from build123d import *

# Parameters (mm, degrees)
F0_W     = 20.5
F0_H     = 4.5
F1_DEPTH = 5
F2_DEPTH = 5
F3_R     = 3
F4_R     = 0.5
F5_DEPTH = 3


with BuildPart() as f1:
    # F0 (on Top) → F1 (new body)
    with BuildSketch(Plane.XY):
        with BuildLine():
            ThreePointArc((4.5, 2.1794494718), (0, -5), (-4.5, 2.1794494718))
            Line((-4.5, 2.1794494718), (-10.5, 2.1794494718))
            Line((-10.5, 2.1794494718), (-11.5394689808, -2.1748499468))
            Line((-11.5394689808, -2.1748499468), (-2, -10))
            Line((-2, -10), (-13.4075078933, -10))
            Line((-13.4075078933, -10), (-16.3915383908, -22.5))
            Line((-16.3915383908, -22.5), (16.3915383908, -22.5))
            Line((16.3915383908, -22.5), (13.4075078933, -10))
            Line((13.4075078933, -10), (2, -10))
            Line((2, -10), (11.5394689808, -2.1748499468))
            Line((11.5394689808, -2.1748499468), (10.5, 2.1794494718))
            Line((10.5, 2.1794494718), (4.5, 2.1794494718))
        make_face()
        with Locations((0, -16.25)):
            Rectangle(F0_W, F0_H, mode=Mode.SUBTRACT)
        with BuildLine():
            Line((4.5, 2.1794494718), (-4.5, 2.1794494718))
            ThreePointArc((-4.5, 2.1794494718), (0, -5), (4.5, 2.1794494718))
        make_face()
    extrude(amount=-F1_DEPTH)

    # F0 (on Top) → F2 (join)
    with BuildSketch(Plane.XY):
        with BuildLine():
            ThreePointArc((4.5, 2.1794494718), (0, -5), (-4.5, 2.1794494718))
            Line((-4.5, 2.1794494718), (-10.5, 2.1794494718))
            Line((-10.5, 2.1794494718), (-11.5394689808, -2.1748499468))
            Line((-11.5394689808, -2.1748499468), (-2, -10))
            Line((-2, -10), (-13.4075078933, -10))
            Line((-13.4075078933, -10), (-16.3915383908, -22.5))
            Line((-16.3915383908, -22.5), (16.3915383908, -22.5))
            Line((16.3915383908, -22.5), (13.4075078933, -10))
            Line((13.4075078933, -10), (2, -10))
            Line((2, -10), (11.5394689808, -2.1748499468))
            Line((11.5394689808, -2.1748499468), (10.5, 2.1794494718))
            Line((10.5, 2.1794494718), (4.5, 2.1794494718))
        make_face()
        with Locations((0, -16.25)):
            Rectangle(F0_W, F0_H, mode=Mode.SUBTRACT)
    extrude(amount=F2_DEPTH)

    # F3
    f3_edges = [f1.edges().sort_by_distance(p)[0] for p in [
        (-16.391538, -22.5, 0),
        (16.391538, -22.5, 0),
        (-10.5, 2.179449, 0),
        (10.5, 2.179449, 0),
        (-2, -10, 0),
        (-13.407508, -10, 0),
        (-11.539469, -2.17485, 0),
        (11.539469, -2.17485, 0),
        (13.407508, -10, 0),
        (2, -10, 0),
    ]]
    fillet(f3_edges, radius=F3_R)

    # F4
    f4_edges = [f1.edges().sort_by_distance(p)[0] for p in [
        (0, -5, 5),
    ]]
    fillet(f4_edges, radius=F4_R)

    # F5 (cut): a face of the model
    f5_faces = [f1.faces().sort_by_distance(p)[0] for p in [
        (0, -1.0065762803, 0),
    ]]
    extrude(f5_faces, amount=-F5_DEPTH, mode=Mode.SUBTRACT)


solid = f1.part
Design review of the part built by this model. Coordinates are the model's own, in mm. A direction names the side the tool comes from. Round coordinates to 2 decimals unless told otherwise and drop trailing zeros. Order: outer loops, then holes, each group sorted by start corner. A loop starts at its lowest first (then second) coordinate and runs counter-clockwise, first axis right, second up.
1) Consider section C-C (x = 0). State the section outline as (y, z) points, plus the area to 3 significant figures.
The answers:
outline: (-22.5, -5) - (-18.5, -5) - (-18.5, 5) - (-22.5, 5) - close; (-14, -5) - (2.18, -5) - (2.18, -3) - (-5, -3) - (-5, 4.5) arc R0.5 ccw to (-5.5, 5) - (-14, 5) - close
area: 144 mm2
2) Consider section B-B (x = -6). State the section outline as (y, z) points.
The answers:
outline: (-22.5, -5) - (-18.5, -5) - (-18.5, 5) - (-22.5, 5) - close; (-14, -5) - (2.18, -5) - (2.18, 5) - (-14, 5) - close
3) Draft analysis for pull direction Y (two halves, no side actions). For faces 1 (the cylindrical face through (0, -5, 1)), 2 (the cylindrical face through (-14.92, -21.39, 0.07)), 3 (the flat face through (0, -22.5, 0)), 4 (the cylindrical face through (10.01, 1.52, -0.07)), state which applies: released by +Y, released by -Y, zero draft, split by the parting line, or undercut.
The answers:
face 1: undercut
face 2: split by the parting line
face 3: released by -Y
face 4: released by +Y
4) Machinability: for faces 5 (the flat face through (-9.3, -4.01, -0.07)), 6 (the flat face through (-14.722, -15.508, -0.07)), 7 (the flat face through (0, -18.5, 0)), which of the approach directions +Z, -Z, +X, -X, +Y, -Y give a long, thin tool a straight path to every point of the face, cutting with its end or side? Answer none if there is none.
The answers:
face 5: +Z, -Z, -X
face 6: +Z, -Z, -X, +Y
face 7: +Z, -Z
5) Consider section A-A (z = 3.75). State the section outline as (x, y) points, plus the area to 3 significant figures.
The answers:
outline: (-15.51, -18.8) arc R3 ccw to (-12.59, -22.5) - (12.59, -22.5) arc R3 ccw to (15.51, -18.8) - (13.96, -12.3) arc R3 ccw to (11.04, -10) - (10.39, -10) arc R3 cw to (8.48, -4.68) - (10.09, -3.37) arc R3 ccw to (11.1, -0.35) - (11.05, -0.12) arc R3 ccw to (8.13, 2.18) - (4.5, 2.18) arc R5 cw (long way) to (-4.5, 2.18) - (-8.13, 2.18) arc R3 ccw to (-11.05, -0.12) - (-11.1, -0.35) arc R3 ccw to (-10.09, -3.37) - (-8.48, -4.68) arc R3 cw to (-10.39, -10) - (-11.04, -10) arc R3 ccw to (-13.96, -12.3) - close; hole (-10.25, -18.5) - (10.25, -18.5) - (10.25, -14) - (-10.25, -14) - close
area: 438 mm2
6) Clearance check with flat-ended pins moving along their axes: pin 1 Ø1.5 at (y, z) = (-11.5, 1.5) entering from +X; pin 2 Ø1.3 at (y, z) = (-16.5, -2) entering from +X; pin 3 Ø3.5 at (x, y) = (1, -1.5) entering from +Z. State where each tip first meets the part, or that it passes through.
The answers:
pin 1: stops at x = 13.94
pin 2: stops at x = 15.11
pin 3: stops at z = -3
7) Consider section D-D (y = -6.75). State the section outline as (x, z) points, plus the area to 3 significant figures.
The answers:
outline: (-7.4, -5) - (7.4, -5) - (7.4, 5) - (-7.4, 5) - close
area: 148 mm2
8) For L1, parallel to Y at x = 0, z = 2.25; L2, parallel to Y at x = 2, z = -4; L3, parallel to Z at x = -1.5, y = -1.5, list the stretches that pass through material, from the lowest coordinate up.
The answers:
L1: y = -22.5 to -18.5, -14 to -5
L2: y = -22.5 to -18.5, -14 to 2.18
L3: z = -5 to -3
